Could you check a few things on this model? Use its own coordinates, in mm. Face numbers are marked on the shaded views. A direction names the side the tool comes from. Round coordinates to 2 decimals unless told otherwise and drop trailing zeros. Order: outer loops, then holes, each group sorted by start corner. A loop starts at its lowest first (then second) coordinate and runs counter-clockwise, first axis right, second up.
```python
from build123d import *

# Parameters (mm, degrees)
BOSS_EXTRUDE1_DEPTH = 10
SKETCH2_R           = 3.25
CUT_EXTRUDE1_DEPTH  = 6
SKETCH3_W           = 41
SKETCH3_H           = 40
BOSS_EXTRUDE2_DEPTH = 23.5
SKETCH6_W           = 40
SKETCH6_H           = 22.5
CUT_EXTRUDE3_DEPTH  = 39
SKETCH7_W           = 8
SKETCH7_H           = 22.5
BOSS_EXTRUDE3_DEPTH = 32
SKETCH8_R           = 0.325
CUT_EXTRUDE4_DEPTH  = 6
SKETCH9_W           = 4.992378119
SKETCH9_H           = 3.003564519
CUT_EXTRUDE5_DEPTH  = 55


with BuildPart() as part:
    # Sketch1 → Boss-Extrude1 (new body)
    with BuildSketch(Plane.XY):
        with BuildLine():
            Line((-69.937444572, 18.545911552), (50.062555428, 18.545911552))
            ThreePointArc((50.062555428, 18.545911552), (70.062555428, -1.454088448), (50.062555428, -21.454088448))
            Line((50.062555428, -21.454088448), (-69.937444572, -21.454088448))
            ThreePointArc((-69.937444572, -21.454088448), (-89.937444572, -1.454088448), (-69.937444572, 18.545911552))
        make_face()
    extrude(amount=BOSS_EXTRUDE1_DEPTH)

    # Sketch2 → Cut-Extrude1 (cut)
    with BuildSketch(Plane.XY.offset(10)):
        with Locations((-69.937444572, -1.454088448)):
            Circle(SKETCH2_R)
    extrude(amount=-CUT_EXTRUDE1_DEPTH, mode=Mode.SUBTRACT)

    # Sketch3 → Boss-Extrude2 (add)
    with BuildSketch(Plane(origin=(0, 0, 0), x_dir=(-1, 0, 0), z_dir=(0, 0, -1))):
        with Locations((-29.444527942, -1.79966235)):
            Rectangle(SKETCH3_W, SKETCH3_H)
    extrude(amount=BOSS_EXTRUDE2_DEPTH)

    # Sketch6 → Cut-Extrude3 (cut)
    with BuildSketch(Plane(origin=(0, 18.20033765, 0), x_dir=(1, 0, 0), z_dir=(0, 1, 0))):
        with Locations((29.465316663, 11.681829122)):
            Rectangle(SKETCH6_W, SKETCH6_H)
    extrude(amount=-CUT_EXTRUDE3_DEPTH, mode=Mode.SUBTRACT)

    # Sketch7 → Boss-Extrude3 (add)
    with BuildSketch(Plane(origin=(0, -20.79966235, 0), x_dir=(1, 0, 0), z_dir=(0, 1, 0))):
        with Locations((13.465316663, 11.681829122)):
            Rectangle(SKETCH7_W, SKETCH7_H)
        with Locations((45.465316663, 11.681829122)):
            Rectangle(SKETCH7_W, SKETCH7_H)
    extrude(amount=BOSS_EXTRUDE3_DEPTH)

    # Sketch8 → Cut-Extrude4 (cut)
    with BuildSketch(Plane(origin=(0, 11.20033765, 0), x_dir=(1, 0, 0), z_dir=(0, 1, 0))):
        with Locations(Location((45.488062991, 17.306829122, 0), (0, 0, 270))):
            Circle(SKETCH8_R)
        with Locations(Location((45.488062991, 6.056829122, 0), (0, 0, 270))):
            Circle(SKETCH8_R)
        with Locations(Location((13.505340173, 17.306829122, 0), (0, 0, 270))):
            Circle(SKETCH8_R)
        with Locations(Location((13.505340173, 6.056829122, 0), (0, 0, 270))):
            Circle(SKETCH8_R)
    extrude(amount=-CUT_EXTRUDE4_DEPTH, mode=Mode.SUBTRACT)

    # Sketch9 → Cut-Extrude5 (cut)
    with BuildSketch(Plane(origin=(0, 0, -23.5), x_dir=(-1, 0, 0), z_dir=(0, 0, -1))):
        with Locations((-29.444527942, 14.360774469)):
            Rectangle(SKETCH9_W, SKETCH9_H)
    extrude(amount=-CUT_EXTRUDE5_DEPTH, mode=Mode.SUBTRACT)


solid = part.part
```
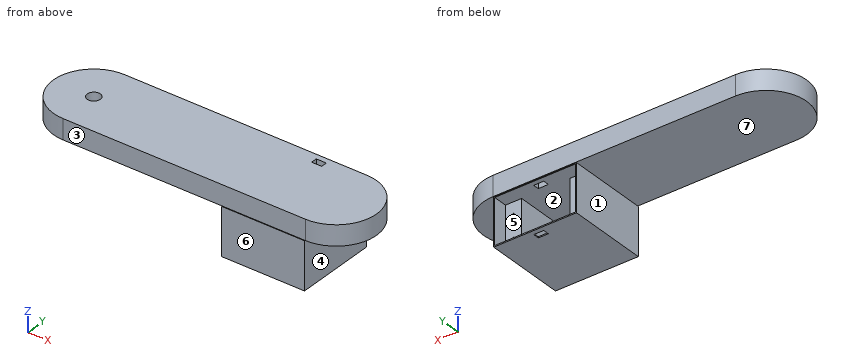
Q1. Imagine slicing it at B-B, the plane z = -11. Please give me the cut outline in (x, y), then the cut area to 3 significant figures.
Q2. For P1, Ø4, axis at x = 45, z = -10, coming from the +Y side; P2, Ø6, axis at x = -69.94, y = -1.45, coming from the -Z side; P3, Ø5, axis at x = 24, z = -4, coming from the +Y side; P4, Ø6, axis at x = 45, z = -1.5, coming from the +Y side, each with a flat end and sliding along its axis, tell me the tip position at first contact or that it passes through.
Q3. We'd pull the mould along Z, two halves only. Please class the marked faces 5, 6 and 7: released by +Z, released by -Z, zero draft, split by the parting line, or undercut.
Q4. Imagine slicing it at A-A, the plane y = -8.5. Please give me the cut outline in (x, z).
Q5. Imagine slicing it at C-C, the plane x = -52. Please give me the cut outline in (y, z), then the cut area to 3 significant figures.
Q6. Imagine slicing it at D-D, the plane z = 6.5. Please give me the cut outline in (x, y), then the cut area to 3 significant figures.
Q7. For the marked faces 1, 2, 3 and 4, which set-ups out of +Z, -Z, +X, -X, +Y, -Y let a thin tool reach every point of the face, with its end or its side?
Q8. I need wall thicknesses on L1, parallel to X at y = 9, z = -6; L2, parallel to X at y = -16, z = -13; L3, parallel to X at y = 14.5, z = -13. Which ranges of each line are inside material? Lowest first, please.
Filled in:
1. outline: (8.94, -21.8) - (49.94, -21.8) - (49.94, 18.2) - (49.47, 18.2) - (49.47, 11.2) - (41.47, 11.2) - (41.47, -20.8) - (17.47, -20.8) - (17.47, 11.2) - (9.47, 11.2) - (9.47, 18.2) - (8.94, 18.2) - close
1. area: 592 mm2
2. P1: stops at y = 11.2
2. P2: stops at z = 0
2. P3: stops at y = -20.8
2. P4: stops at y = 18.55
3. face 5: undercut
3. face 6: zero draft
3. face 7: released by -Z
4. outline: (-88.66, 0) - (8.94, 0) - (8.94, -23.5) - (49.94, -23.5) - (49.94, 0) - (68.78, 0) - (68.78, 10) - (-88.66, 10) - close; hole (17.47, -22.93) - (41.47, -22.93) - (41.47, -0.43) - (17.47, -0.43) - close
5. outline: (-21.45, 0) - (18.55, 0) - (18.55, 10) - (-21.45, 10) - close
5. area: 400 mm2
6. outline: (-69.94, -21.45) - (50.06, -21.45) arc R20 ccw to (50.06, 18.55) - (-69.94, 18.55) arc R20 ccw to start; hole circle Ø6.5 at (-69.94, -1.45); hole (26.95, 12.86) - (31.94, 12.86) - (31.94, 15.86) - (26.95, 15.86) - close
6. area: 6,010 mm2
7. face 1: -Z, -X, +Y, -Y
7. face 2: +Y
7. face 3: +Z, +X, -X, -Y
7. face 4: -Z, +X, +Y, -Y
8. L1: x = 8.94 to 13.19, 13.83 to 17.47, 41.47 to 45.17, 45.81 to 49.94
8. L2: x = 8.94 to 17.47, 41.47 to 49.94
8. L3: x = 8.94 to 9.47, 49.47 to 49.94
